Build history of the part. All positions in model axes, mm. A direction names the side the tool comes from. Round coordinates to 2 decimals unless told otherwise and drop trailing zeros. Order: outer loops, then holes, each group sorted by start corner. A loop starts at its lowest first (then second) coordinate and runs counter-clockwise, first axis right, second up. Notation, with made-up numbers: M 74,40 L 128,40 A27 cw 128,76 Z; hole C 68,3 d5. An arc over 180 degrees is marked long. One line per item, written item: value. Start each with the question number.
Item 1: Pin check, flat tips, straight feed: pin 1 (1.4 mm diameter, centred on x = -6.5, y = 7.5, fed in from -Z); pin 2 (1.3 mm diameter, centred on x = -13, z = -38.5, fed in from +Y); pin 3 (1.4 mm diameter, centred on x = -12.5, y = 7.5, fed in from +Z). Stop position of each tip, or through.
Item 2: Band-saw the part on B-B, the plane y = 6.75. Write the cut outline in (x, z).
Item 3: Band-saw the part on A-A, the plane x = -19.05. Give the number of separate pieces and of enclosed holes in the cut face, then the cut area to 3 significant figures.
Item 4: Tool access for faces 5 (the flat face through (-13, 6.35, -15)), 6 (the flat face through (-25.4, 3, -20)): list every direction of +Z, -Z, +X, -X, +Y, -Y with a clear straight run to the whole face (end or side of a thin tool).
Item 5: Two-plate mould, pull along Z, no slides. Class faces 1 (the flat face through (-13, 7, -35.7)), 2 (the flat face through (-13, 7, -29.705)), 3 (the cylindrical face through (-8.04, 3.131, -9.145)), 4 (the flat face through (-13, 6.35, -38)): +Z half, -Z half, draft (parallel to the pull), parting line (faces both ways), or undercut.
Item 6: Band-saw the part on C-C, the plane z = -34. Write the cut outline in (x, y), then the cut area to 3 significant figures.
Item 7: Probe L1, parallel to Z at x = -19.05, y = 1.5 (1 decimal); L2, parallel to X at y = 5.75, z = -32; L3, parallel to Z at x = -20.75, y = 5.75 (3 decimals). List the from-to ranges inside material, lowest first.
Autodesk Inventor part; units mm, degrees
ref_plane "YZ Plane" through (0, 0, 0) normal (1, 0, 0) x (0, 1, 0)
ref_plane "XZ Plane" through (0, 0, 0) normal (0, 1, 0) x (-1, 0, 0)
ref_plane "XY Plane" through (0, 0, 0) normal (0, 0, 1) x (1, 0, 0)
sketch "Sketch1" plane through (0, 0, 0) normal (0, 1, 0) x (-1, 0, 0)
  line L0 (0, 0) -> (25.4, 0)
  line L1 (25.4, 0) -> (25.4, -40.005)
  line L2 (25.4, -40.005) -> (0, -40.005)
  line L3 (0, -40.005) -> (0, 0)
  dimension "d0" = 40.005
  dimension "d1" = 25.4
extrude "Extrusion1" add sketch "Sketch1" along normal blind 6.35
sketch "Sketch2" plane through (0, 6.35, 0) normal (0, 1, 0) x (1, 0, 0)
  line L0 (-25.4, 40.005) -> (-25.4, 0)
  line L1 (0, 0) -> (0, 40.005)
  line L2 (-25.4, 35.6997) -> (0, 35.6997)
  line L3 (0, 35.6997) -> (0, 29.7053)
  line L4 (0, 29.7053) -> (-25.4, 29.7053)
  line L5 (-25.4, 29.7053) -> (-25.4, 35.6997)
  line L6 (-25.4, 32.7025) -> (0, 32.7025) construction
  line L7 (-25.4, 7.3025) -> (0, 7.3025)
  line L8 (-25.4, 0) -> (0, 0)
  line L9 (0, 40.005) -> (-25.4, 40.005)
  line L10 (-25.4, 29.7053) -> (0, 29.7053)
  line L11 (0, 29.7053) -> (0, 35.6997)
  line L12 (0, 35.6997) -> (-25.4, 35.6997)
  line L13 (-25.4, 35.6997) -> (-25.4, 29.7053)
  line L14 (-12.7, 35.6997) -> (-12.7, 29.7053) construction
  line L15 (-6.35, 7.3025) -> (-6.35, 40.005) construction
  line L16 (-19.05, 7.3025) -> (-19.05, 40.005) construction
  point P0 (-12.7, 32.7025)
  dimension "d4" = 5.9944
  dimension "d5" = 25.4
  dimension "d6" = 7.3025
  dimension "d7" = 40.005
  dimension "d8" = 12.7
  dimension "d9" = 25.4
  dimension "d10" = 6.35
  dimension "d23" = 12.7
extrude "Extrusion2" add sketch "Sketch2" along normal blind 5.715 contours L2 L1 L4 L0
hole "Hole1" at (-19.05, 6.35, -7.3025) at (-6.35, 6.35, -7.3025) direction (0, -1, 0) diameter 5 end through all
sketch "Sketch3" plane through (0, 0, 0) normal (1, 0, 0) x (0, 0, -1)
  line L0 (29.7053, 12.065) -> (35.6997, 12.065)
  line L1 (40.005, 0) -> (0, 0)
  line L2 (40.005, 0) -> (40.005, 6.35)
  line L3 (35.6997, 6.35) -> (40.005, 6.35)
  line L4 (35.6997, 6.35) -> (35.6997, 12.065)
  line L5 (29.7053, 12.065) -> (35.6997, 12.065)
  line L6 (29.7053, 6.35) -> (29.7053, 12.065)
  line L7 (0, 6.35) -> (29.7053, 6.35)
  line L8 (0, 0) -> (0, 6.35)
  line L9 (29.7053, 6.35) -> (35.6997, 6.35)
  line L10 (35.6997, 6.35) -> (35.6997, 8.128)
  line L11 (35.6997, 6.35) -> (35.6997, 12.065)
  line L12 (35.6997, 8.128) -> (29.7053, 8.128)
  line L13 (29.7053, 8.128) -> (29.7053, 6.35)
  line L14 (29.7053, 8.128) -> (29.7053, 12.065)
  line L15 (29.7053, 12.065) -> (35.6997, 12.065)
  line L16 (35.6997, 12.065) -> (35.6997, 8.128)
  dimension "d20" = 1.778
extrude "Extrusion3" cut sketch "Sketch3" against normal through all contours L0 L4 L12 L6
ref_plane "Work Plane1" through (-12.7, 0, -40.005) normal (-1, 0, 0) x (0, 0, 1)
sketch "Sketch4" plane through (0, 8.128, -29.7053) normal (0, 1, 0) x (1, 0, 0)
  circle A0 centre (-6.35, -22.4028) radius 2.5
  circle A1 centre (-19.05, -22.4028) radius 2.5
  line L0 (0, 5.9944) -> (0, 0)
  point P0 (0, -29.7053)
  point P1 (-6.35, 2.9972)
  point P2 (-19.05, 2.9972)
  point P3 (0, 2.9972)
hole "Hole2" at (-6.35, 8.128, -32.7025) at (-19.05, 8.128, -32.7025) direction (0, -1, 0) diameter 5 end through all
equation "\"d6\" = -0.5 * d5 + 0.5 * d7"
equation "\"d10\" = -0.5 * d8 + 0.5 * d9"
equation "\"d24\" = d13"
properties part number "slider manual tension v1"
Output:
1. pin 1: stops at z = -35.7
1. pin 2: stops at y = 6.35
1. pin 3: stops at z = -29.71
2. outline: M -25.4,-35.7 L 0,-35.7 L 0,-29.71 L -25.4,-29.71 Z; hole C -19.05,-32.7 d5; hole C -6.35,-32.7 d5
3. separate pieces: 3
3. enclosed holes: 0
3. area: 192 mm²
4. face 5: +Z, +X, -X, +Y
4. face 6: +Z, -Z, -X, +Y, -Y
5. face 1: -Z half
5. face 2: +Z half
5. face 3: undercut
5. face 4: draft
6. outline: M -25.4,0 L -21.19,0 L -21.19,8.13 L -25.4,8.13 Z; M -16.91,0 L -8.49,0 L -8.49,8.13 L -16.91,8.13 Z; M -4.21,0 L 0,0 L 0,8.13 L -4.21,8.13 Z
6. area: 137 mm²
7. L1: z = -40 to -35.2, -30.2 to -9.8, -4.8 to 0
7. L2: x = -25.4 to -21.45, -16.65 to -8.75, -3.95 to 0
7. L3: z = -40.005 to -34.536, -30.869 to -9.136, -5.469 to 0
